Verification items for the finished model (mm, model axes). Face numbers are marked on the shaded views. Coordinates: 2 decimals unless noted, no trailing zeros. Order: outer loops, then holes, each group sorted by start corner. A loop starts at its lowest first (then second) coordinate and runs counter-clockwise, first axis right, second up. Notation, with made-up numbers: (72.5, 32.5) -> (131.5, 32.5) arc R17 ccw to (131.5, 39.5) -> close; hole circle Ø3 at (70, 47). An arc over 180 degrees is marked (long way). Write item = value, one per line. Start each with the question number.
1. Thickness scan on line 1 along Y through (x, z) = (6.3, 0.65); line 2 along X through (y, z) = (14.5, 0.8); line 3 along X through (y, z) = (12, 0.5). Record the ranges inside material, lowest first. Write a range as from..to.
2. Go/stop test with a flat-tipped pin: P1, Ø4, axis at x = 8.5, y = 4.5, coming from the -Z side. Record where the tip stops, or that it passes through.
3. Cross-section at B-B on x = 6.3. Record the cut outline in (y, z), plus the area to 3 significant figures.
4. Cross-section at A-A on z = 0.75. Give the number of separate pieces and of enclosed holes in the cut face, plus the area to 3 significant figures.
5. Cross-section at D-D on y = 24. Record the cut outline in (x, z).
6. Release check for a two-part mould opening along Z. For the marked faces 1 and 2 record: +Z half, -Z half, draft (parallel to the pull), parting line (faces both ways), or undercut.
7. Cross-section at C-C on y = 12.7. Record the cut outline in (x, z), plus the area to 3 significant figures.
from build123d import *
from OCP.BRepFilletAPI import BRepFilletAPI_MakeFillet

# Parameters (mm, degrees)
SKETCH1_R           = 3.302
SKETCH1_R_2         = 4.5
BOSS_EXTRUDE1_DEPTH = 0.9144
FILLET2_R           = 7.5
FILLET2_R_2         = 3.5


with BuildPart() as part:
    # Sketch1 → Boss-Extrude1 (new body)
    # profile 1 of 2: a face of its own
    with BuildSketch(Plane.XY):
        Polygon((26.3, 25.4), (37.6, 25.4), (37.6, 0), (0, 0), (0, 25.4), (11.3, 25.4), (11.3, 37.4), (26.3, 37.4), align=None)
        with Locations((31.3, 12.7)):
            Circle(SKETCH1_R, mode=Mode.SUBTRACT)
        with Locations((6.3, 12.7)):
            Circle(SKETCH1_R, mode=Mode.SUBTRACT)
        with Locations((18.8, 29.9)):
            Circle(SKETCH1_R_2, mode=Mode.SUBTRACT)
    # profile 2 of 2: a face of its own
    with BuildSketch(Plane.XY):
        with Locations((18.8, 29.9)):
            Circle(SKETCH1_R_2)
    extrude(amount=BOSS_EXTRUDE1_DEPTH)

    # Fillet2
    fillet2_edges_1 = [part.edges().sort_by_distance(p)[0] for p in [
        (11.3, 37.4, 0.4572),
        (26.3, 37.4, 0.4572),
    ]]
    fillet2_edges_2 = [part.edges().sort_by_distance(p)[0] for p in [
        (11.3, 25.4, 0.4572),
        (0, 25.4, 0.4572),
        (0, 0, 0.4572),
        (37.6, 25.4, 0.4572),
        (26.3, 25.4, 0.4572),
        (37.6, 0, 0.4572),
    ]]
    fillet2 = BRepFilletAPI_MakeFillet(part.part.solid().wrapped)
    for e in fillet2_edges_1:
        fillet2.Add(FILLET2_R - 0.0001, e.wrapped)
    for e in fillet2_edges_2:
        fillet2.Add(FILLET2_R_2 - 0.0001, e.wrapped)
    add(Compound.cast(fillet2.Shape()), mode=Mode.REPLACE)  # a hair under: the kernel refuses the full size


solid = part.part
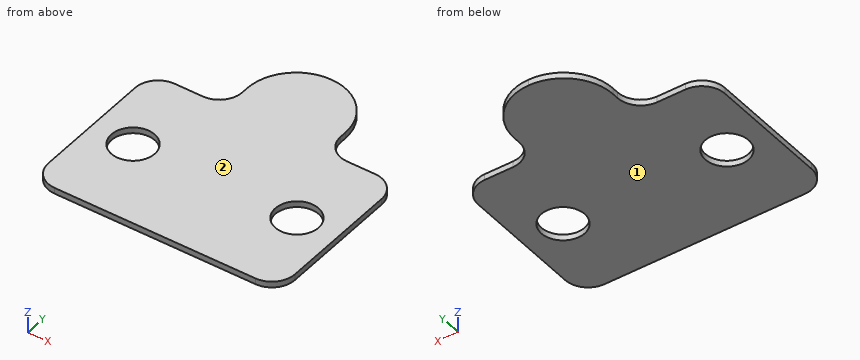
Worked out:
q1.line_1 = 0..9.4, 16..25.4
q1.line_2 = 0..3.53, 9.07..28.53, 34.07..37.6
q1.line_3 = 0..3.07, 9.53..28.07, 34.53..37.6
q2.P1 = 0
q3.outline = (0, 0) -> (9.4, 0) -> (9.4, 0.91) -> (0, 0.91) -> close; (16, 0) -> (25.4, 0) -> (25.4, 0.91) -> (16, 0.91) -> close
q3.area = 17.2 mm²
q4.separate_pieces = 1
q4.enclosed_holes = 2
q4.area = 1,040 mm²
q5.outline = (0.7, 0) -> (36.9, 0) -> (36.9, 0.91) -> (0.7, 0.91) -> close
q6.face_1 = -Z half
q6.face_2 = +Z half
q7.outline = (0, 0) -> (3, 0) -> (3, 0.91) -> (0, 0.91) -> close; (9.6, 0) -> (28, 0) -> (28, 0.91) -> (9.6, 0.91) -> close; (34.6, 0) -> (37.6, 0) -> (37.6, 0.91) -> (34.6, 0.91) -> close
q7.area = 22.3 mm²
